Design review of the part built by this model. Coordinates are the model's own, in mm. A direction names the side the tool comes from. Round coordinates to 2 decimals unless told otherwise and drop trailing zeros. Order: outer loops, then holes, each group sorted by start corner. A loop starts at its lowest first (then second) coordinate and runs counter-clockwise, first axis right, second up. Notation, with made-up numbers: (36, 38.5) - (66, 38.5) arc R21 ccw to (66, 61.5) - close; hole circle Ø11 at (74.25, 33.5). An arc over 180 degrees is marked (long way). Use CSV: the item, a comma, the result in double quotes.
from build123d import *

# Parameters (mm, degrees)
SKETCH_1_R          = 14
SKETCH_1_R_2        = 1.5
EXTRUDE_1_DEPTH     = 2
CUT_EXTRUDE_1_DEPTH = 20.899748742
EXTRUDE_4_DEPTH     = 1
SKETCH_6_R          = 7
SKETCH_6_R_2        = 3.1
EXTRUDE_5_DEPTH     = 5
EXTRUDE_6_DEPTH     = 1
SKETCH_8_W          = 8
SKETCH_8_H          = 2
EXTRUDE_7_DEPTH     = 5
SKETCH_9_R          = 1.6
CUT_EXTRUDE_3_DEPTH = 24.108440017
EXTRUDE_8_DEPTH     = 2
SKETCH_11_W         = 12.041493288
SKETCH_11_H         = 2
CUT_EXTRUDE_4_DEPTH = 5
SKETCH_12_R         = 20
SKETCH_12_R_2       = 3.1
EXTRUDE_9_DEPTH     = 2
SKETCH_13_R         = 2.3
CUT_EXTRUDE_5_DEPTH = 2
CUT_EXTRUDE_START   = -1
CUT_EXTRUDE_6_DEPTH = 1
FILLET_1_R          = 3
FILLET_2_R          = 1.5


with BuildPart() as part:
    # 草图1 → 凸台-拉伸1 (new body)
    with BuildSketch(Plane.XY):
        Circle(SKETCH_1_R)
        with Locations((-7.071067812, 7.071067812)):
            Circle(SKETCH_1_R_2, mode=Mode.SUBTRACT)
        with Locations((7.071067812, 7.071067812)):
            Circle(SKETCH_1_R_2, mode=Mode.SUBTRACT)
        with Locations((-7.071067812, -7.071067812)):
            Circle(SKETCH_1_R_2, mode=Mode.SUBTRACT)
        with Locations((7.071067812, -7.071067812)):
            Circle(SKETCH_1_R_2, mode=Mode.SUBTRACT)
    extrude(amount=EXTRUDE_1_DEPTH)

    # 草图2 → 切除-拉伸1 (cut, through all)
    with BuildSketch(Plane(origin=(0, 0, 0), x_dir=(-1, 0, 0), z_dir=(0, 0, -1))):
        with BuildLine():
            ThreePointArc((-2.683281573, 3.1), (-4.1, 0), (-2.683281573, -3.1))
            Line((-2.683281573, -3.1), (2.683281573, -3.1))
            ThreePointArc((2.683281573, -3.1), (4.1, 0), (2.683281573, 3.1))
            Line((2.683281573, 3.1), (-2.683281573, 3.1))
        make_face()
    extrude(amount=-CUT_EXTRUDE_1_DEPTH, mode=Mode.SUBTRACT)

    # 草图3 → 凸台-拉伸4 (add)
    with BuildSketch(Plane(origin=(0, 0, 0), x_dir=(-1, 0, 0), z_dir=(0, 0, -1))):
        Polygon((0, 3.1), (3.7, 3.1), (3.7, 7.1), (-3.7, 7.1), (-3.7, 3.1), align=None)
    extrude(amount=EXTRUDE_4_DEPTH)

    # 草图6 → 凸台-拉伸5 (add)
    with BuildSketch(Plane(origin=(0, 0, -1), x_dir=(-1, 0, 0), z_dir=(0, 0, -1))):
        with Locations(Location((0, 0, 0), (0, 0, 121.908982735))):
            Circle(SKETCH_6_R)
        with Locations(Location((0, 0, 0), (0, 0, 90))):
            Circle(SKETCH_6_R_2, mode=Mode.SUBTRACT)
    extrude(amount=EXTRUDE_5_DEPTH)

    # 草图7 → 凸台-拉伸6 (add)
    with BuildSketch(Plane(origin=(0, 0, -6), x_dir=(-1, 0, 0), z_dir=(0, 0, -1))):
        with BuildLine():
            Line((-2.5, 3.1), (-2.5, 6.538348415))
            ThreePointArc((-2.5, 6.538348415), (0, 7), (2.5, 6.538348415))
            Line((2.5, 6.538348415), (2.5, 3.1))
            Line((2.5, 3.1), (-2.5, 3.1))
        make_face()
    extrude(amount=EXTRUDE_6_DEPTH)

    # 草图8 → 凸台-拉伸7 (add)
    with BuildSketch(Plane(origin=(0, 0, -6), x_dir=(-1, 0, 0), z_dir=(0, 0, -1))):
        with Locations((9.447401339, 2)):
            Rectangle(SKETCH_8_W, SKETCH_8_H)
        with Locations((9.447401339, -2)):
            Rectangle(SKETCH_8_W, SKETCH_8_H)
    extrude(amount=-EXTRUDE_7_DEPTH)

    # 草图9 → 切除-拉伸3 (cut, through all)
    with BuildSketch(Plane(origin=(0, 3, 0), x_dir=(1, 0, 0), z_dir=(0, 1, 0))):
        with Locations(Location((-10.8, 4, 0), (0, 0, 180))):
            Circle(SKETCH_9_R)
    extrude(amount=-CUT_EXTRUDE_3_DEPTH, mode=Mode.SUBTRACT)

    # 草图10 → 凸台-拉伸8 (add)
    with BuildSketch(Plane(origin=(0, 0, -7), x_dir=(-1, 0, 0), z_dir=(0, 0, -1))):
        with BuildLine():
            Line((-2.5, 6.538348415), (-2.5, 3.1))
            ThreePointArc((-2.5, 3.1), (0, -3.98246155), (2.5, 3.1))
            Line((2.5, 3.1), (2.5, 6.538348415))
            ThreePointArc((2.5, 6.538348415), (0, 7), (-2.5, 6.538348415))
        make_face()
    extrude(amount=EXTRUDE_8_DEPTH)

    # 草图11 → 切除-拉伸4 (cut)
    with BuildSketch(Plane(origin=(0, 0, -6), x_dir=(-1, 0, 0), z_dir=(0, 0, -1))):
        with Locations((7.426654695, 0)):
            Rectangle(SKETCH_11_W, SKETCH_11_H)
    extrude(amount=-CUT_EXTRUDE_4_DEPTH, mode=Mode.SUBTRACT)

    # 草图12 → 凸台-拉伸9 (add)
    with BuildSketch(Plane.XY.offset(2)):
        Circle(SKETCH_12_R)
        Circle(SKETCH_12_R_2, mode=Mode.SUBTRACT)
    extrude(amount=-EXTRUDE_9_DEPTH)

    # 草图13 → 切除-拉伸5 (cut)
    with BuildSketch(Plane.XY.offset(2)):
        with Locations((10.253048327, 10.253048327)):
            Circle(SKETCH_13_R)
        with Locations((-10.253048327, 10.253048327)):
            Circle(SKETCH_13_R)
        with Locations((-10.253048327, -10.253048327)):
            Circle(SKETCH_13_R)
        with Locations((10.253048327, -10.253048327)):
            Circle(SKETCH_13_R)
    extrude(amount=-CUT_EXTRUDE_5_DEPTH, mode=Mode.SUBTRACT)

    # 草图14 → 切除-拉伸6 (cut)
    with BuildSketch(Plane(origin=(0, 0, -1), x_dir=(-1, 0, 0), z_dir=(0, 0, -1)).offset(CUT_EXTRUDE_START)):
        with BuildLine():
            Line((-4.590882623, 5.284297185), (-4.590882623, 9.738638689))
            Line((-4.590882623, 9.738638689), (4.724825977, 9.738638689))
            Line((4.724825977, 9.738638689), (4.724825977, 5.164883298))
            ThreePointArc((4.724825977, 5.164883298), (0.089722487, 6.999424967), (-4.590882623, 5.284297185))
        make_face()
    extrude(amount=CUT_EXTRUDE_6_DEPTH, mode=Mode.SUBTRACT)

    # 圆角1
    fillet_1_edges = [part.edges().sort_by_distance(p)[0] for p in [
        (0, 7, -9),
    ]]
    fillet(fillet_1_edges, radius=FILLET_1_R)

    # 圆角2
    fillet_2_edges = [part.edges().sort_by_distance(p)[0] for p in [
        (-13.447401339, -2, -1),
        (-13.447401339, -2, -6),
        (-13.447401339, 2, -1),
        (-13.447401339, 2, -6),
    ]]
    fillet(fillet_2_edges, radius=FILLET_2_R)


solid = part.part
1) To check wall thickness, follow L1, parallel to Y at x = 0, z = -4.9; L2, parallel to Z at x = 5.5, y = 15.5; L3, parallel to Z at x = 6, y = 3.5. State the ranges of each line that lie inside material, in increasing order. Write a range as from..to.
Data:
L1,"y = -7..-3.1, 3.1..7"
L2,"z = 0..2"
L3,"z = -6..-1, 0..2"
2) The part is to be moulded in two halves that separate along Y. For faces 5 (the face through (-13.447, 2, -4)), 6 (the face through (-8, 1, -4)), 7 (the face through (0, 3.1, -6.5)), say which applies: +Y half, -Y half, draft (parallel to the pull), parting line (faces both ways), or undercut.
Data:
face 5,"draft"
face 6,"undercut"
face 7,"-Y half"
3) We need section D-D (y = -11). Give the boundary of the cut face in (x, z).
Data:
outline,"(-16.7, 0) - (-12.43, 0) - (-12.43, 2) - (-16.7, 2) - close; (-8.08, 0) - (8.08, 0) - (8.08, 2) - (-8.08, 2) - close; (12.43, 0) - (16.7, 0) - (16.7, 2) - (12.43, 2) - close"
4) We need section C-C (x = -10.8). Give the boundary of the cut face in (y, z).
Data:
outline,"(-16.83, 0) - (-12.49, 0) - (-12.49, 2) - (-16.83, 2) - close; (-8.02, 0) - (8.02, 0) - (8.02, 2) - (-8.02, 2) - close; (-3, -6) - (-1, -6) - (-1, -5.6) - (-3, -5.6) - close; (-3, -2.4) - (-1, -2.4) - (-1, -1) - (-3, -1) - close; (1, -6) - (3, -6) - (3, -5.6) - (1, -5.6) - close; (1, -2.4) - (3, -2.4) - (3, -1) - (1, -1) - close; (12.49, 0) - (16.83, 0) - (16.83, 2) - (12.49, 2) - close"
5) We need section B-B (y = -6.5). Give the boundary of the cut face in (x, z), then the cut area to 3 significant figures.
Data:
outline,"(-18.91, 0) - (18.91, 0) - (18.91, 2) - (-18.91, 2) - close; (-2.6, -6) - (2.6, -6) - (2.6, -1) - (-2.6, -1) - close"
area,"102 mm2"
6) Insertion check: pin 1 Ø1.9 at (x, z) = (-10.8, -4) entering from -Y; pin 2 Ø4 at (x, z) = (6.5, -4) entering from -Y; pin 3 Ø5 at (x, z) = (-14.5, -5.5) entering from -Y; pin 4 Ø4 at (x, z) = (-5.5, -3.5) entering from +Y. Each pin has a flat end and moves straight along its axis. Give the tip position at first contact, or say it passes through.
Data:
pin 1,"passes through"
pin 2,"stops at y = -5.36"
pin 3,"stops at y = -3"
pin 4,"stops at y = 6.06"
7) We need section A-A (y = 0). Give the boundary of the cut face in (x, z).
Data:
outline,"(-20, 0) - (-3.1, 0) - (-3.1, 2) - (-20, 2) - close; (-3.98, -9) - (3.98, -9) - (3.98, -7) - (-3.98, -7) - close; (3.1, -6) - (7, -6) - (7, -1) - (3.1, -1) - close; (3.1, 0) - (20, 0) - (20, 2) - (3.1, 2) - close"
8) For faces 1 (the face through (-3.7, 4.5, -0.5)), 2 (the face through (3.7, 4.5, -0.5)), 3 (the face through (-8, -1, -4)), 4 (the face through (-2.5, 4, -7)), list the 3-axis set-ups (+Z, -Z, +X, -X, +Y, -Y) from which the entire face can be reached by the end or side of a thin tool; tool diameter is ignored.
Data:
face 1,"-X, +Y, -Y"
face 2,"+X, +Y, -Y"
face 3,"-X"
face 4,"-Z, -X, +Y"
